The model under review builds one solid part; all positions refer to its coordinate system, in mm. A direction names the side the tool comes from. Coordinates: 2 decimals unless noted, no trailing zeros. Loops run counter-clockwise (first coordinate to the right, second up) from the corner with the lowest first, then second, coordinate; pieces in that order, holes last. Notation, with made-up numbers: M -8,61 L 8,61 A19 ccw 8,80 Z; hole C -16,64.25 d5. An arc over 180 degrees is marked long. Use one line per item in the form item = value.
```python
from build123d import *

# Parameters (mm, degrees)
SKETCH3_R               = 5
CUT_EXTRUDE1_DEPTH      = 13.5000001
CUT_EXTRUDE1_DEPTH_BACK = 433.5000001


with BuildPart() as part:
    # Sweep-Thin1: sweep along a path in Sketch1
    with BuildLine(Plane(origin=(0, 0, 0), x_dir=(1, 0, 0), z_dir=(0, 1, 0))) as sweep_thin1_path:
        Line((0, 0), (-410, 0))
        ThreePointArc((-410, 0), (-438.284271247, 11.715728753), (-450, 40))
        Line((-450, 40), (-450, 380))
        ThreePointArc((-450, 380), (-438.284271247, 408.284271247), (-410, 420))
        Line((-410, 420), (0, 420))
    # Sketch2 → Sweep-Thin1 (sweep)
    with BuildSketch(Plane(origin=(0, 0, 0), x_dir=(0, 0, -1), z_dir=(1, 0, 0))):
        with BuildLine():
            Line((4.5, 12.5), (-4.5, 12.5))
            ThreePointArc((-4.5, 12.5), (-10.156854249, 10.156854249), (-12.5, 4.5))
            Line((-12.5, 4.5), (-12.5, -4.5))
            ThreePointArc((-12.5, -4.5), (-10.156854249, -10.156854249), (-4.5, -12.5))
            Line((-4.5, -12.5), (4.5, -12.5))
            ThreePointArc((4.5, -12.5), (10.156854249, -10.156854249), (12.5, -4.5))
            Line((12.5, -4.5), (12.5, 4.5))
            ThreePointArc((12.5, 4.5), (10.156854249, 10.156854249), (4.5, 12.5))
        make_face()
        with BuildLine():
            Line((4.5, 9.5), (-4.5, 9.5))
            ThreePointArc((-4.5, 9.5), (-8.035533906, 8.035533906), (-9.5, 4.5))
            Line((-9.5, 4.5), (-9.5, -4.5))
            ThreePointArc((-9.5, -4.5), (-8.035533906, -8.035533906), (-4.5, -9.5))
            Line((-4.5, -9.5), (4.5, -9.5))
            ThreePointArc((4.5, -9.5), (8.035533906, -8.035533906), (9.5, -4.5))
            Line((9.5, -4.5), (9.5, 4.5))
            ThreePointArc((9.5, 4.5), (8.035533906, 8.035533906), (4.5, 9.5))
        make_face(mode=Mode.SUBTRACT)
    sweep(path=sweep_thin1_path.line)

    # Sketch3 → Cut-Extrude1 (cut, two sides)
    with BuildSketch(Plane.XY) as cut_extrude1_sk:
        with Locations((-50, 0)):
            Circle(SKETCH3_R)
    extrude(amount=CUT_EXTRUDE1_DEPTH, mode=Mode.SUBTRACT)
    extrude(cut_extrude1_sk.sketch, amount=-CUT_EXTRUDE1_DEPTH_BACK, mode=Mode.SUBTRACT)


solid = part.part
```
1. Machinability: for faces 1 (the face through (-446.71, -0.06, -2.47)), 2 (the face through (-447, 9.5, -209)), 3 (the face through (-429.66, 0.06, -399.23)), which of the approach directions +Z, -Z, +X, -X, +Y, -Y give a long, thin tool a straight path to every point of the face, cutting with its end or side? Answer none if there is none.
Response values:
face_1 = +Z, -X, +Y, -Y
face_2 = none
face_3 = +X, +Y, -Y
2. Add section A-A (x = -232). Count the separate pieces of the cut face and the enclosed holes in it, then the cut area to 3 significant figures.
Response values:
separate_pieces = 2
enclosed_holes = 2
area = 461 mm^2
3. Wall thickness on line 1 along Z through (x, y) = (-372.5, 5); line 2 along X through (y, z) = (1.5, -147.5); line 3 along Z through (x, y) = (-220.5, 5.25): over which ranges is each line inside the solid? List them lowest first. Write a range as from..to.
Response values:
line_1 = -432.48..-429.47, -410.53..-407.52, -12.48..-9.47, 9.47..12.48
line_2 = -462.5..-459.5, -440.5..-437.5
line_3 = -432.46..-429.44, -410.56..-407.54, -12.46..-9.44, 9.44..12.46
4. The part is to be moulded in two halves that separate along Y. For faces 4 (the face through (0, 0, -11)), 5 (the face through (-55, 0, 11)), 6 (the face through (-447, -12.5, -209)), say which applies: pulls with the +Y half, pulls with the -Y half, needs draft (parallel to the pull), parting line crosses it, or undercut.
Response values:
face_4 = needs draft
face_5 = undercut
face_6 = pulls with the -Y half
5. Add section B-B (z = -83.5). State the section outline as (x, y) points, then the cut area to 3 significant figures.
Response values:
outline = M -462.5,-4.5 A8 ccw -454.5,-12.5 L -445.5,-12.5 A8 ccw -437.5,-4.5 L -437.5,4.5 A8 ccw -445.5,12.5 L -454.5,12.5 A8 ccw -462.5,4.5 Z; hole M -459.5,-4.5 A5 ccw -454.5,-9.5 L -445.5,-9.5 A5 ccw -440.5,-4.5 L -440.5,4.5 A5 ccw -445.5,9.5 L -454.5,9.5 A5 ccw -459.5,4.5 Z
area = 231 mm^2
6. Insertion check: P1, Ø2, axis at y = 6.5, z = -95.5, coming from the +X side; P2, Ø8, axis at y = 9.5, z = -96, coming from the -X side; P3, Ø2.5, axis at y = -1.5, z = -201.5, coming from the +X side. Each pin has a flat end and moves straight along its axis. Give the tip position at first contact, or say it passes through.
Response values:
P1 = -437.56
P2 = -462.44
P3 = -437.5
